from build123d import *

# Parameters (mm, degrees)
SKETCH2_R           = 1.755
BOSS_EXTRUDE1_DEPTH = 6
SKETCH3_W           = 9.5
SKETCH3_H           = 29.5
BOSS_EXTRUDE2_DEPTH = 3
SKETCH4_R           = 2
CUT_EXTRUDE1_DEPTH  = 22.624638725
FILLET1_R           = 2


with BuildPart() as part:
    # Sketch2 → Boss-Extrude1 (new body)
    with BuildSketch(Plane.XY):
        with BuildLine():
            Line((-4.75, 6), (-4.75, 0))
            ThreePointArc((-4.75, 0), (0, -4.75), (4.75, 0))
            Line((4.75, 0), (4.75, 6))
            Line((4.75, 6), (-4.75, 6))
        make_face()
        Circle(SKETCH2_R, mode=Mode.SUBTRACT)
    extrude(amount=BOSS_EXTRUDE1_DEPTH)

    # Sketch3 → Boss-Extrude2 (add)
    with BuildSketch(Plane(origin=(0, 6, 0), x_dir=(1, 0, 0), z_dir=(0, 1, 0))):
        with Locations((0, -1.25)):
            Rectangle(SKETCH3_W, SKETCH3_H)
    extrude(amount=BOSS_EXTRUDE2_DEPTH)

    # Sketch4 → Cut-Extrude1 (cut, through all)
    with BuildSketch(Plane(origin=(0, 9, 0), x_dir=(1, 0, 0), z_dir=(0, 1, 0))):
        with Locations(Location((0, -11.5, 0), (0, 0, 270))):
            Circle(SKETCH4_R)
        with Locations(Location((0, 9, 0), (0, 0, 270))):
            Circle(SKETCH4_R)
    extrude(amount=-CUT_EXTRUDE1_DEPTH, mode=Mode.SUBTRACT)

    # Fillet1
    fillet1_edges = [part.edges().sort_by_distance(p)[0] for p in [
        (4.75, 7.5, -13.5),
        (-4.75, 7.5, -13.5),
        (-4.75, 7.5, 16),
        (4.75, 7.5, 16),
    ]]
    fillet(fillet1_edges, radius=FILLET1_R)


solid = part.part
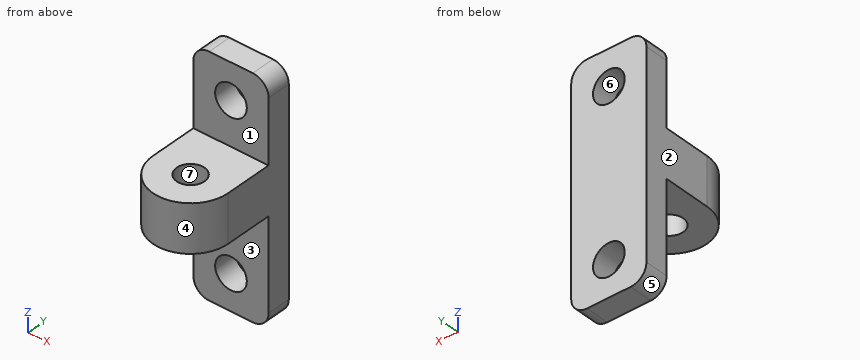
Here's how the part is built. I have some questions about the finished solid (model axes, mm). Face numbers are marked on the shaded views. A direction names the side the tool comes from. Round coordinates to 2 decimals unless told otherwise and drop trailing zeros. Write each loop counter-clockwise with the first axis right and the second up, starting at its lowest first coordinate (ties: lowest second). Pieces come first, ordered by that corner, then holes.
1. Suppose I cut it at A-A (x = 0). List the corners of the cut face in (y, z) for me (3 decimals), and give its area (3 significant figures).
2. For the marked faces 1, 2 and 3, which set-ups out of +Z, -Z, +X, -X, +Y, -Y let a thin tool reach every point of the face, with its end or its side?
3. Will these pins go through, and if not, where does the flat tip stop? pin 1 Ø4 at (x, z) = (-0.5, -8) entering from -Y; pin 2 Ø5 at (x, z) = (0, 11.5) entering from +Y; pin 3 Ø5 at (x, y) = (1.5, -0.5) entering from +Z; pin 4 Ø3 at (x, y) = (0, 0) entering from -Z.
4. Suppose I cut it at B-B (z = -9). List the corners of the cut face in (x, y) for me, and give its area (3 significant figures).
5. Suppose I cut it at D-D (x = 3.25). List the corners of the cut face in (y, z) for me.
6. Suppose I cut it at C-C (y = 7.5). List the corners of the cut face in (x, z) for me, and give its area (3 significant figures).
7. If we mould it in two halves opening along X, with no side actions, what happens to the marked faces 4, 5, 6 and 7? For each: released by +X, released by -X, zero draft, split by the parting line, or undercut.
8. I need wall thicknesses on L1, parallel to X at y = 8.15, z = 11.5; L2, parallel to Y at x = 1.25, z = -11; L3, parallel to Z at x = 1, y = 2. Which ranges of each line are inside material? Lowest first, please.
Answer sheet:
1. outline: (-4.75, 0) - (-1.755, 0) - (-1.755, 6) - (-4.75, 6) - close; (1.755, 0) - (6, 0) - (6, -7) - (9, -7) - (9, 9.5) - (6, 9.5) - (6, 6) - (1.755, 6) - close; (6, -13.5) - (9, -13.5) - (9, -11) - (6, -11) - close; (6, 13.5) - (9, 13.5) - (9, 16) - (6, 16) - close
1. area: 108 mm2
2. face 1: +Z, +X, -X, -Y
2. face 2: +Z, -Z, -X, +Y, -Y
2. face 3: -Z, +X, -X, -Y
3. pin 1: stops at y = 6
3. pin 2: stops at y = 9
3. pin 3: stops at z = 6
3. pin 4: passes through
4. outline: (-4.75, 6) - (-2, 6) - (-2, 9) - (-4.75, 9) - close; (2, 6) - (4.75, 6) - (4.75, 9) - (2, 9) - close
4. area: 16.5 mm2
5. outline: (-3.46, 0) - (6, 0) - (6, -13.44) - (9, -13.44) - (9, 15.94) - (6, 15.94) - (6, 6) - (-3.46, 6) - close
6. outline: (-4.75, -11.5) arc R2 ccw to (-2.75, -13.5) - (2.75, -13.5) arc R2 ccw to (4.75, -11.5) - (4.75, 14) arc R2 ccw to (2.75, 16) - (-2.75, 16) arc R2 ccw to (-4.75, 14) - close; hole circle Ø4 at (0, -9); hole circle Ø4 at (0, 11.5)
6. area: 252 mm2
7. face 4: split by the parting line
7. face 5: released by -X
7. face 6: undercut
7. face 7: undercut
8. L1: x = -4.75 to -2, 2 to 4.75
8. L2: y = 6 to 9
8. L3: z = 0 to 6
